Design review of the part shown in the three views and the two pictorial views. Dimensions are in mm from the part's minimum x, y and z. A direction names the side the tool comes from. Coordinates: 2 decimals unless noted, no trailing zeros. Loops run counter-clockwise (first coordinate to the right, second up) from the corner with the lowest first, then second, coordinate; pieces in that order, holes last. Notation, with made-up numbers: (60, -31.75) -> (88, -31.75) arc R19 ccw to (88, -12.75) -> close; hole circle Ø9 at (-25, 6.5). An arc over 180 degrees is marked (long way). One line per item, written item: value. Start each with the question number.
1. Add section A-A on x = 45. Write out the cut boundary in (y, z).
2. Insertion check: pin 1 (3 mm diameter, centred on x = 35, z = 16.5, fed in from +Y); pin 2 (10 mm diameter, centred on x = 3.5, z = 15, fed in from -Y); pin 3 (8 mm diameter, centred on y = 15.5, z = 31.5, fed in from +X); pin 4 (1.5 mm diameter, centred on x = 12.5, y = 16.5, fed in from +Z). Each pin has a flat end and moves straight along its axis. Give the tip position at first contact, or say it passes through.
3. Machinability: for the marked faces 1, 2, 3, 4 and 5, which of the approach directions +Z, -Z, +X, -X, +Y, -Y give a long, thin tool a straight path to every point of the face, cutting with its end or side? Answer none if there is none.
4. For probe 1 along X at (y, z) = (30, 35); probe 2 along Z at (x, y) = (5, 29.65); probe 3 along X at (y, z) = (28, 17), list the stretches that pass through material, from the lowest coordinate up.
5. Add section B-B on z = 20. Write out the cut boundary in (x, y), plus the area to 3 significant figures.
6. Add section C-C on y = 25.5. Write out the cut boundary in (x, z), plus the area to 3 significant figures.
7. Add section D-D on z = 35. Write out the cut boundary in (x, y).
8. Draft analysis for pull direction X (two halves, no side actions). For the marked faces 6, 7 and 8, state which applies: pulls with the +X half, pulls with the -X half, needs draft (parallel to the pull), parting line crosses it, or undercut.
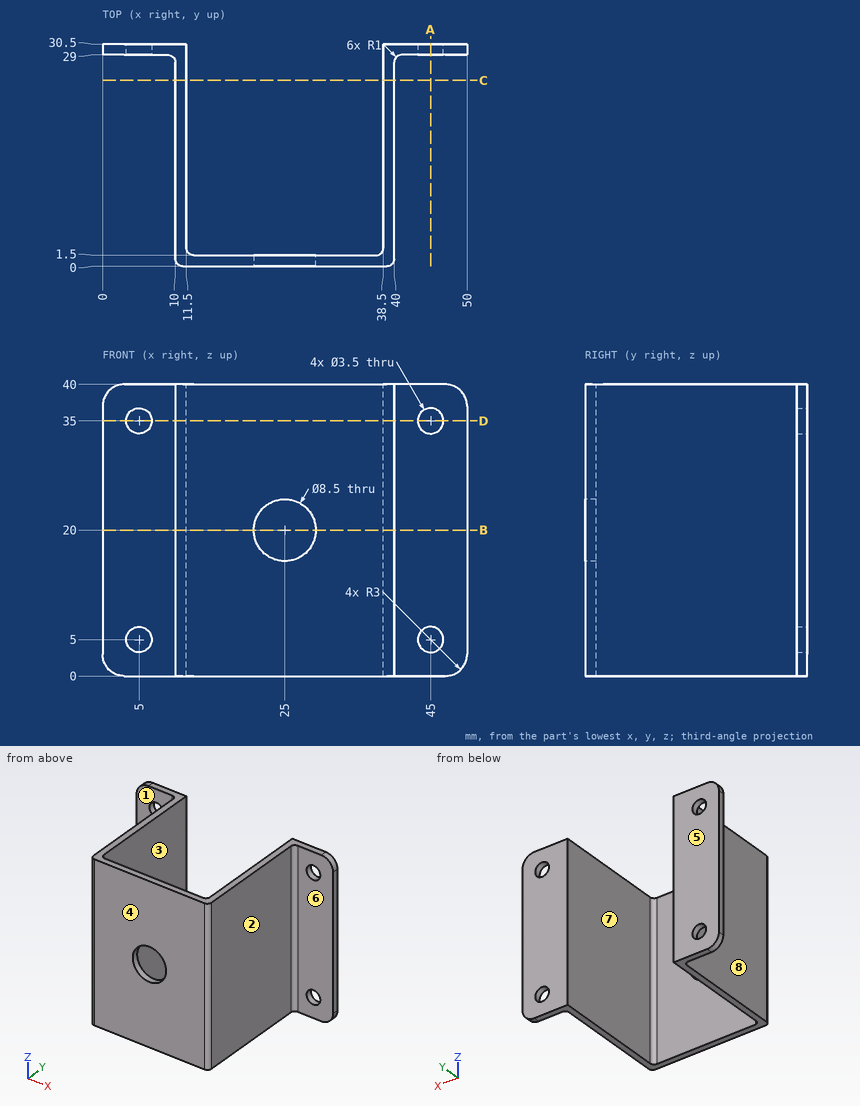
Worked answers:
1. outline: (29, 0) -> (30.5, 0) -> (30.5, 3.25) -> (29, 3.25) -> close; (29, 6.75) -> (30.5, 6.75) -> (30.5, 33.25) -> (29, 33.25) -> close; (29, 36.75) -> (30.5, 36.75) -> (30.5, 40) -> (29, 40) -> close
2. pin 1: stops at y = 1.5
2. pin 2: stops at y = 29
2. pin 3: stops at x = 40
2. pin 4: passes through
3. face 1: +Z, -Z, -X, -Y
3. face 2: +Z, -Z, +X, -Y
3. face 3: +Z, -Z, +Y
3. face 4: +Z, -Z, +X, -X, -Y
3. face 5: +Z, -Z, +X, -X, +Y
4. probe 1: x = 0 to 3.25, 6.75 to 11.5, 38.5 to 43.25, 46.75 to 50
4. probe 2: z = 0 to 3.25, 6.75 to 33.25, 36.75 to 40
4. probe 3: x = 10 to 11.5, 38.5 to 40
5. outline: (0, 29) -> (9, 29) arc R1 cw to (10, 28) -> (10, 1) arc R1 ccw to (11, 0) -> (20.75, 0) -> (20.75, 1.5) -> (12.5, 1.5) arc R1 cw to (11.5, 2.5) -> (11.5, 30.5) -> (0, 30.5) -> close; (29.25, 0) -> (39, 0) arc R1 ccw to (40, 1) -> (40, 28) arc R1 cw to (41, 29) -> (50, 29) -> (50, 30.5) -> (38.5, 30.5) -> (38.5, 2.5) arc R1 cw to (37.5, 1.5) -> (29.25, 1.5) -> close
5. area: 150 mm²
6. outline: (10, 0) -> (11.5, 0) -> (11.5, 40) -> (10, 40) -> close; (38.5, 0) -> (40, 0) -> (40, 40) -> (38.5, 40) -> close
6. area: 120 mm²
7. outline: (0, 29) -> (3.25, 29) -> (3.25, 30.5) -> (0, 30.5) -> close; (6.75, 29) -> (9, 29) arc R1 cw to (10, 28) -> (10, 1) arc R1 ccw to (11, 0) -> (39, 0) arc R1 ccw to (40, 1) -> (40, 28) arc R1 cw to (41, 29) -> (43.25, 29) -> (43.25, 30.5) -> (38.5, 30.5) -> (38.5, 2.5) arc R1 cw to (37.5, 1.5) -> (12.5, 1.5) arc R1 cw to (11.5, 2.5) -> (11.5, 30.5) -> (6.75, 30.5) -> close; (46.75, 29) -> (50, 29) -> (50, 30.5) -> (46.75, 30.5) -> close
8. face 6: needs draft
8. face 7: undercut
8. face 8: pulls with the -X half
